For this review, take the finished solid that the model builds, in its own axes (mm). A direction names the side the tool comes from. Give positions to 0.01 mm unless a question says otherwise; leave off trailing zeros. Write each loop counter-clockwise with the first axis right and the second up, starting at its lowest first coordinate (ties: lowest second). Pieces come first, ordered by that corner, then holes. Notation, with made-up numbers: (67, 36.25) -> (83, 36.25) arc R31 cw to (83, 69.25) -> close; hole circle Ø2 at (25, 47.5). An arc over 180 degrees is marked (long way). Return JSON: item names as keys, results as strings.
from build123d import *

# Parameters (mm, degrees)
F0_W     = 20
F0_H     = 30
F1_DEPTH = 30
F2_DEPTH = 10
F3_SIZE  = 10


with BuildPart() as f1:
    # F0 (on Top) → F1 (new body)
    with BuildSketch(Plane.XY):
        with Locations((10, 15)):
            Rectangle(F0_W, F0_H)
    extrude(amount=F1_DEPTH)

    # F0 (on Top) → F2 (join)
    with BuildSketch(Plane.XY):
        Polygon((20, 30), (20, 0), (30, 0), (40, 10), (40, 40), (0, 40), (0, 30), align=None)
    extrude(amount=F2_DEPTH)

    # F3
    f3_edges = [f1.edges().sort_by_distance(p)[0] for p in [
        (10, 0, 30),
    ]]
    chamfer(f3_edges, length=F3_SIZE)


solid = f1.part
1. Add section A-A, the plane x = 6. State the section outline as (y, z) points, plus the area to 3 significant figures.
Results found:
{"outline": "(0, 0) -> (40, 0) -> (40, 10) -> (30, 10) -> (30, 30) -> (10, 30) -> (0, 20) -> close", "area": "950 mm²"}
2. Add section D-D, the plane y = 27. State the section outline as (x, z) points.
Results found:
{"outline": "(0, 0) -> (40, 0) -> (40, 10) -> (20, 10) -> (20, 30) -> (0, 30) -> close"}
3. For pin 1 (3 mm diameter, centred on y = 4.5, z = 20, fed in from +X); pin 2 (10 mm diameter, centred on x = 29, y = 6.5, fed in from +Z); pin 3 (4 mm diameter, centred on x = 18, z = 21.5, fed in from +Y), all flat-tipped, find the tip position at first contact; note any pin that passes through.
Results found:
{"pin 1": "stops at x = 20", "pin 2": "stops at z = 10", "pin 3": "stops at y = 30"}
4. Add section B-B, the plane y = 4. State the section outline as (x, z) points, plus the area to 3 significant figures.
Results found:
{"outline": "(0, 0) -> (34, 0) -> (34, 10) -> (20, 10) -> (20, 24) -> (0, 24) -> close", "area": "620 mm²"}
5. For faces 1 (the flat face through (10, 30, 20)), 2 (the flat face through (35, 5, 5)), 3 (the flat face through (20, 15, 20)), list the 3-axis set-ups (+Z, -Z, +X, -X, +Y, -Y) from which the entire face can be reached by the end or side of a thin tool; tool diameter is ignored.
Results found:
{"face 1": "+Z, +X, -X, +Y", "face 2": "+Z, -Z, +X, -Y", "face 3": "+Z, +X, +Y, -Y"}
6. To check wall thickness, follow probe 1 along Z at (x, y) = (27.5, 5.5); probe 2 along X at (y, z) = (28, 15); probe 3 along Y at (x, z) = (10, 14.25). State the ranges of each line that lie inside material, in increasing order.
Results found:
{"probe 1": "z = 0 to 10", "probe 2": "x = 0 to 20", "probe 3": "y = 0 to 30"}
7. Add section C-C, the plane z = 23.5. State the section outline as (x, y) points, plus the area to 3 significant figures.
Results found:
{"outline": "(0, 3.5) -> (20, 3.5) -> (20, 30) -> (0, 30) -> close", "area": "530 mm²"}
